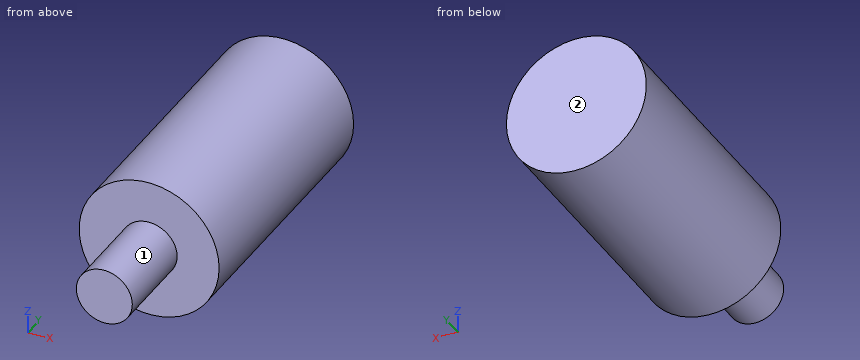
```python
from build123d import *

# Parameters (mm, degrees)
CYLINDER1217_R     = 1.6
CYLINDER1217_DEPTH = 15
CYLINDER1202_R     = 4
CYLINDER1202_DEPTH = 15


with BuildPart() as cylinder1217:
    # Cylinder1217 → Cylinder1217 (new body)
    with BuildSketch(Plane(origin=(480, 87, 115), x_dir=(1, 0, 0), z_dir=(0, -1, 0))):
        Circle(CYLINDER1217_R)
    extrude(amount=CYLINDER1217_DEPTH)


with BuildPart() as fusion248002050129:
    # Cylinder1202 → Cylinder1202 (new body)
    with BuildSketch(Plane(origin=(480, 92, 115), x_dir=(1, 0, 0), z_dir=(0, -1, 0))):
        Circle(CYLINDER1202_R)
    extrude(amount=CYLINDER1202_DEPTH)

    # Fusion248002050129: union Cylinder1217
    add(cylinder1217.part)


with BuildPart() as fusion248002050129_1:
    # Fusion248002050129 placement: moved
    add(fusion248002050129.part.moved(Location((0.5, 0, 0))))


solid = fusion248002050129_1.part
```
Work out the finished part from the listing and answer in its coordinate system (mm). Face numbers are marked on the shaded views. A direction names the side the tool comes from. Round coordinates to 2 decimals unless told otherwise and drop trailing zeros. Loops run counter-clockwise (first coordinate to the right, second up) from the corner with the lowest first, then second, coordinate; pieces in that order, holes last.
(1) The part is cut by section D-D, the plane y = 85. Give the vertices of the cut face in (x, z).
Computed values:
outline: circle Ø8 at (480.5, 115)
(2) The part is cut by section B-B, the plane x = 480.5. Give the vertices of the cut face in (y, z), and give its area (3 significant figures).
Computed values:
outline: (72, 113.4) - (77, 113.4) - (77, 111) - (92, 111) - (92, 119) - (77, 119) - (77, 116.6) - (72, 116.6) - close
area: 136 mm2
(3) The part is cut by section A-A, the plane z = 115. Give the vertices of the cut face in (x, y), and give its area (3 significant figures).
Computed values:
outline: (476.5, 77) - (478.9, 77) - (478.9, 72) - (482.1, 72) - (482.1, 77) - (484.5, 77) - (484.5, 92) - (476.5, 92) - close
area: 136 mm2
(4) Find the intervals of material crossed by L1, parallel to Y at x = 478.75, z = 118.5; L2, parallel to Z at x = 480, y = 84.75; L3, parallel to Z at x = 477.25, y = 77.5, in increasing order.
Computed values:
L1: y = 77 to 92
L2: z = 111.03 to 118.97
L3: z = 112.67 to 117.33
(5) For the marked faces 1 and 2, determine the directions among +Z, -Z, +X, -X, +Y, -Y from which every point of the face is accessible in a straight line to the end or side of a thin tool.
Computed values:
face 1: -Y
face 2: +Z, -Z, +X, -X, +Y
(6) Each of these flat-tipped pins is pushed along its axis until it touches: P1, Ø4, axis at y = 79.5, z = 114, coming from the -X side; P2, Ø1.5, axis at x = 481.5, y = 86.5, coming from the +Z side; P3, Ø1, axis at x = 478, y = 80, coming from the -Z side. Where does it stop, or does it pass through?
Computed values:
P1: stops at x = 476.5
P2: stops at z = 118.99
P3: stops at z = 111.54
(7) The part is cut by section C-C, the plane y = 76. Give the vertices of the cut face in (x, z), and give its area (3 significant figures).
Computed values:
outline: circle Ø3.2 at (480.5, 115)
area: 8.04 mm2
